Can you work these out from the model? Positions are in its coordinate system, mm. Coordinates: 2 decimals unless noted, no trailing zeros. Order: outer loops, then holes, each group sorted by start corner. A loop starts at its lowest first (then second) coordinate and runs counter-clockwise, first axis right, second up. Notation, with made-up numbers: (72, -35.75) -> (87, -35.75) arc R24 ccw to (87, -15.75) -> close; hole circle Ø9 at (34.25, 86.5). An arc over 180 degrees is marked (long way). Use a Markdown table: item, result. Add a question column.
1. Suppose I cut it at B-B, the plane z = -2.25. List the corners of the cut face in (x, y) for me, then the cut area to 3 significant figures.
2. For pin 1 Ø2 at (y, z) = (62.5, -4.5) entering from -X; pin 2 Ø4 at (x, y) = (-2, 228) entering from -Z, each with a flat end and sliding along its axis, tell me the tip position at first contact or that it passes through.
3. Suppose I cut it at A-A, the plane y = 110. List the corners of the cut face in (x, z) for me.
4. If I drill on line 1 along Z through (x, y) = (-0.75, 164); line 2 along X through (y, z) = (341, -1.5); line 3 along X through (y, z) = (458, 0.5), over which ranges is the centre line in solid material (lowest first)? Write a range as from..to.
Autodesk Inventor part; units mm, degrees
ref_plane "YZ Plane" through (0, 0, 0) normal (1, 0, 0) x (0, 1, 0)
ref_plane "XZ Plane" through (0, 0, 0) normal (0, 1, 0) x (-1, 0, 0)
ref_plane "XY Plane" through (0, 0, 0) normal (0, 0, 1) x (1, 0, 0)
sketch "Sketch1" plane through (0, 0, 0) normal (0, 1, 0) x (-1, 0, 0)
  circle A0 centre (0, 0) radius 6.35
  line L0 (3.1132, 5.5345) -> (6.3496, 0.0712)
  line L1 (6.3496, 0.0712) -> (3.2364, -5.4633)
  line L2 (3.2364, -5.4633) -> (-3.1132, -5.5345)
  line L3 (-3.1132, -5.5345) -> (-6.3496, -0.0712)
  line L4 (-6.3496, -0.0712) -> (-3.2364, 5.4633)
  line L5 (-3.2364, 5.4633) -> (3.1132, 5.5345)
  dimension "d0" = 12.7
extrude "Extrusion1" add sketch "Sketch1" along normal blind 508 contours L1 L2 L3 L4 L5 L0
properties part number "SuperHexagon"
Worked out:
| question | item | result |
|---|---|---|
| 1 | outline | (-5.04, 0) -> (5.06, 0) -> (5.06, 508) -> (-5.04, 508) -> close |
| 1 | area | 5,130 mm² |
| 2 | pin 1 | stops at x = -4.34 |
| 2 | pin 2 | stops at z = -5.5 |
| 3 | outline | (-6.35, 0.07) -> (-3.24, -5.46) -> (3.11, -5.53) -> (6.35, -0.07) -> (3.24, 5.46) -> (-3.11, 5.53) -> close |
| 4 | line 1 | z = -5.49..5.51 |
| 4 | line 2 | x = -5.47..5.5 |
| 4 | line 3 | x = -6.1..6.03 |
